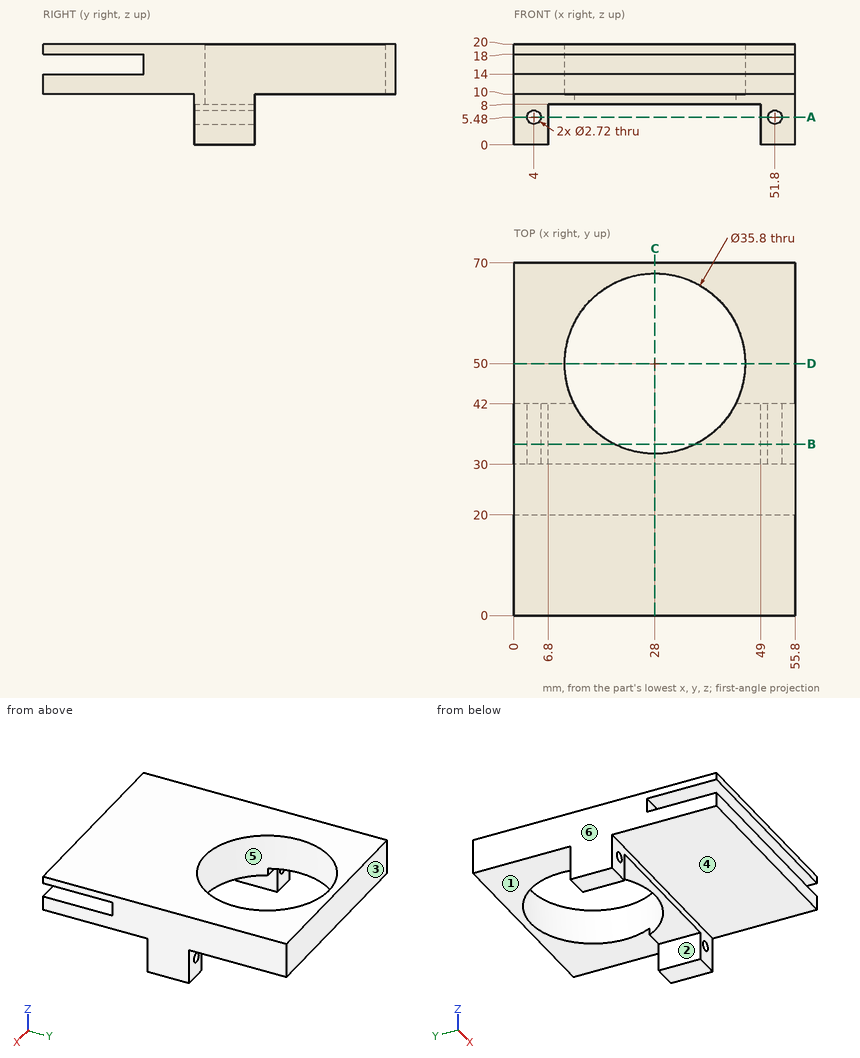
Can you work these out from the drawing? Everything is in mm from the part's minimum corner. A direction names the side the tool comes from. Round coordinates to 2 decimals unless told otherwise and drop trailing zeros. Order: outer loops, then holes, each group sorted by start corner. A loop starts at its lowest first (then second) coordinate and runs counter-clockwise, first axis right, second up.
(1) If we section it at C-C (x = 28): Please give me the cut outline in (y, z).
Results are:
outline: (0, 10) - (30, 10) - (30, 8) - (32.1, 8) - (32.1, 20) - (0, 20) - (0, 18) - (20, 18) - (20, 14) - (0, 14) - close; (67.9, 10) - (70, 10) - (70, 20) - (67.9, 20) - close
(2) On a 3-axis mill with a long thin cutter (end or side, diameter ignored), from which of +Z, -Z, +X, -X, +Y, -Y can I reach the whole of each face in a straight line? I mean the marked faces 1, 2 and 3. Say none if no direction works.
Results are:
face 1: -Z, +X, -X, +Y
face 2: -Z, +Y, -Y
face 3: +Z, -Z, +X, -X, +Y
(3) We'd pull the mould along X, two halves only. Please class the marked faces 4, 5 and 6: +X half, -X half, draft (parallel to the pull), parting line (faces both ways), or undercut.
Results are:
face 4: draft
face 5: undercut
face 6: -X half
(4) If I drill on L1, parallel to X at y = 33.75, z = 5.48; L2, parallel to Z at x = 4, y = 37.5; L3, parallel to Y at x = 28, z = 16.5, over which ranges is the centre line in solid material (lowest first)?
Results are:
L1: x = 0 to 2.64, 5.36 to 6.8, 49 to 50.44, 53.16 to 55.8
L2: z = 0 to 4.12, 6.84 to 20
L3: y = 20 to 32.1, 67.9 to 70
(5) If we section it at D-D (y = 50): Please give me the cut outline in (x, z), plus the area to 3 significant figures.
Results are:
outline: (0, 10) - (10.1, 10) - (10.1, 20) - (0, 20) - close; (45.9, 10) - (55.8, 10) - (55.8, 20) - (45.9, 20) - close
area: 200 mm2
(6) If we section it at A-A (z = 5.48): Please give me the cut outline in (x, y), plus the area to 3 significant figures.
Results are:
outline: (0, 30) - (2.64, 30) - (2.64, 42) - (0, 42) - close; (5.36, 30) - (6.8, 30) - (6.8, 42) - (5.36, 42) - close; (49, 30) - (50.44, 30) - (50.44, 42) - (49, 42) - close; (53.16, 30) - (55.8, 30) - (55.8, 42) - (53.16, 42) - close
area: 97.9 mm2
(7) If we section it at B-B (y = 34): Please give me the cut outline in (x, z).
Results are:
outline: (0, 0) - (6.8, 0) - (6.8, 8) - (19.97, 8) - (19.97, 20) - (0, 20) - close; (36.03, 8) - (49, 8) - (49, 0) - (55.8, 0) - (55.8, 20) - (36.03, 20) - close; hole circle Ø2.72 at (4, 5.48); hole circle Ø2.72 at (51.8, 5.48)
(8) I'm going to push flat-ended pins straight in: pin 1 (3 mm diameter, centred on x = 3.5, z = 7.5, fed in from +Y); pin 2 (3 mm diameter, centred on x = 39.5, z = 5, fed in from -Y) (1 decimal); pin 3 (22.5 mm diameter, centred on x = 14.5, y = 54.5, fed in from -Z); pin 4 (2 mm diameter, centred on x = 34.5, z = 15.5, fed in from -Y). Where does each tip first touch, or does it pass through?
Results are:
pin 1: stops at y = 42
pin 2: passes through
pin 3: stops at z = 10
pin 4: stops at y = 20
